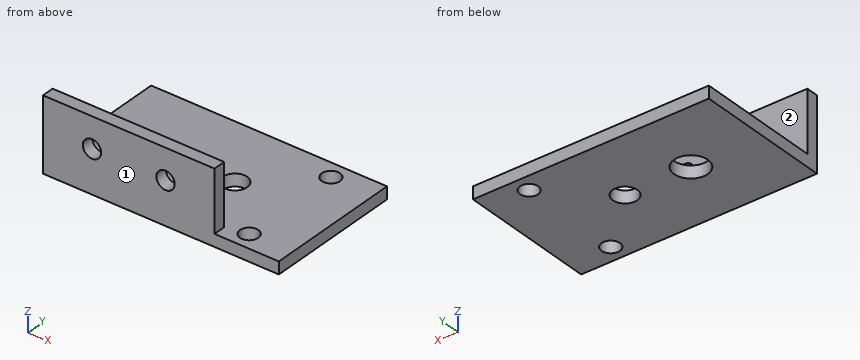
from build123d import *

# Parameters (mm, degrees)
SKETCH1_W           = 38.5
SKETCH1_H           = 22.5
SKETCH1_R           = 2.75
SKETCH1_R_2         = 2
SKETCH1_R_3         = 1.5
BOSS_EXTRUDE1_DEPTH = 2
SKETCH2_W           = 10
SKETCH2_H           = 2
BOSS_EXTRUDE2_DEPTH = 28
SKETCH4_R           = 1.5
CUT_EXTRUDE1_DEPTH  = 5


with BuildPart() as part:
    # Sketch1 → Boss-Extrude1 (new body)
    with BuildSketch(Plane.XY):
        Rectangle(SKETCH1_W, SKETCH1_H)
        with Locations((-7.5, 0)):
            Circle(SKETCH1_R, mode=Mode.SUBTRACT)
        with Locations((3.25, 0)):
            Circle(SKETCH1_R_2, mode=Mode.SUBTRACT)
        with Locations((12.25, -8.5)):
            Circle(SKETCH1_R_3, mode=Mode.SUBTRACT)
        with Locations((12.25, 8.5)):
            Circle(SKETCH1_R_3, mode=Mode.SUBTRACT)
    extrude(amount=BOSS_EXTRUDE1_DEPTH)

    # Sketch2 → Boss-Extrude2 (add)
    with BuildSketch(Plane.ZY.offset(19.25)):
        with Locations((7, -10.25)):
            Rectangle(SKETCH2_W, SKETCH2_H)
    extrude(amount=-BOSS_EXTRUDE2_DEPTH)

    # Sketch4 → Cut-Extrude1 (cut)
    with BuildSketch(Plane(origin=(0, -9.25, 0), x_dir=(1, 0, 0), z_dir=(0, 1, 0))):
        with Locations(Location((-11.25, -7, 0), (0, 0, 270))):  # turned: the seam where the file's is
            Circle(SKETCH4_R)
        with Locations(Location((0.75, -7, 0), (0, 0, 270))):  # turned: the seam where the file's is
            Circle(SKETCH4_R)
    extrude(amount=-CUT_EXTRUDE1_DEPTH, mode=Mode.SUBTRACT)


solid = part.part
Geometry check sheet. Reference: the model listing, model coordinates, mm. Face numbers are marked on the shaded views. A direction names the side the tool comes from. Round coordinates to 2 decimals unless told otherwise and drop trailing zeros. Order: outer loops, then holes, each group sorted by start corner. A loop starts at its lowest first (then second) coordinate and runs counter-clockwise, first axis right, second up. Notation, with made-up numbers: (39, -23) -> (96, -23) arc R23 ccw to (96, 13) -> close; hole circle Ø7 at (30.5, 65). An arc over 180 degrees is marked (long way). Use one line per item in the form item = value.
1. Cross-section at C-C, the plane y = 0. Enter the section's corners in (x, z).
Working result:
outline = (-19.25, 0) -> (-10.25, 0) -> (-10.25, 2) -> (-19.25, 2) -> close; (-4.75, 0) -> (1.25, 0) -> (1.25, 2) -> (-4.75, 2) -> close; (5.25, 0) -> (19.25, 0) -> (19.25, 2) -> (5.25, 2) -> close
2. Cross-section at A-A, the plane y = 8.5. Enter the section's corners in (x, z), plus the area to 3 significant figures.
Working result:
outline = (-19.25, 0) -> (10.75, 0) -> (10.75, 2) -> (-19.25, 2) -> close; (13.75, 0) -> (19.25, 0) -> (19.25, 2) -> (13.75, 2) -> close
area = 71.0 mm^2
3. Go/stop test with flat-tipped pins: pin 1 (3.5 mm diameter, centred on x = 0.75, z = 7, fed in from -Y); pin 2 (11 mm diameter, centred on x = -3, y = -0.5, fed in from +Z); pin 3 (5 mm diameter, centred on x = 3, z = 8.5, fed in from +Y); pin 4 (0.6 mm diameter, centred on y = -10.5, z = 7, fed in from +X). Record where each tip stops, or that it passes through.
Working result:
pin_1 = -11.25
pin_2 = 2
pin_3 = -9.25
pin_4 = 8.75
4. Cross-section at D-D, the plane z = 7.25. Enter the section's corners in (x, y), plus the area to 3 significant figures.
Working result:
outline = (-19.25, -11.25) -> (-12.73, -11.25) -> (-12.73, -9.25) -> (-19.25, -9.25) -> close; (-9.77, -11.25) -> (-0.73, -11.25) -> (-0.73, -9.25) -> (-9.77, -9.25) -> close; (2.23, -11.25) -> (8.75, -11.25) -> (8.75, -9.25) -> (2.23, -9.25) -> close
area = 44.2 mm^2
5. Set-up check for the marked faces 1 and 2: record each of +Z, -Z, +X, -X, +Y, -Y from which the full face is reachable in a straight line by a thin tool's end or side.
Working result:
face_1 = +Z, -Z, +X, -X, -Y
face_2 = +Z, +X, -X, +Y
6. Cross-section at B-B, the plane x = 3.25. Enter the section's corners in (y, z), plus the area to 3 significant figures.
Working result:
outline = (-11.25, 0) -> (-2, 0) -> (-2, 2) -> (-9.25, 2) -> (-9.25, 12) -> (-11.25, 12) -> close; (2, 0) -> (11.25, 0) -> (11.25, 2) -> (2, 2) -> close
area = 57.0 mm^2
7. Scan lines: line 1 along Y through (x, z) = (12.25, 0.9); line 2 along Y through (x, z) = (3.25, 0.7); line 3 along Y through (x, z) = (-7.5, 1.65). Record each from-to range of solid material in increasing order. Write a range as from..to.
Working result:
line_1 = -11.25..-10, -7..7, 10..11.25
line_2 = -11.25..-2, 2..11.25
line_3 = -11.25..-2.75, 2.75..11.25
